Build history of the part. All positions in model axes, mm. A direction names the side the tool comes from. Coordinates: 2 decimals unless noted, no trailing zeros. Order: outer loops, then holes, each group sorted by start corner. A loop starts at its lowest first (then second) coordinate and runs counter-clockwise, first axis right, second up. Notation, with made-up numbers: (46.5, 59) - (102.5, 59) arc R21 ccw to (102.5, 95) - close; hole circle Ø3 at (-35, 7.5). An arc over 180 degrees is marked (long way). One line per item, written item: value.
from build123d import *

# Parameters (mm, degrees)
SKETCH1_W           = 40
SKETCH1_H           = 12.1
BOSS_EXTRUDE1_DEPTH = 3
SKETCH2_W           = 40
SKETCH2_H           = 3
SKETCH2_H_2         = 7
BOSS_EXTRUDE2_DEPTH = 10
SKETCH3_W           = 10.2
SKETCH3_H           = 3.2
CUT_EXTRUDE1_DEPTH  = 44.765397291
SKETCH4_W           = 4
SKETCH4_H           = 8
CUT_EXTRUDE2_DEPTH  = 20
SKETCH5_R           = 4.5
CUT_EXTRUDE3_DEPTH  = 3
FILLET2_R           = 10
FILLET1_R           = 0.4


with BuildPart() as part:
    # Sketch1 → Boss-Extrude1 (new body)
    with BuildSketch(Plane(origin=(0, 0, 0), x_dir=(1, 0, 0), z_dir=(0, 1, 0))):
        with Locations((20, -6.05)):
            Rectangle(SKETCH1_W, SKETCH1_H)
    extrude(amount=BOSS_EXTRUDE1_DEPTH)

    # Sketch2 → Boss-Extrude2 (add)
    with BuildSketch(Plane(origin=(0, 3, 0), x_dir=(1, 0, 0), z_dir=(0, 1, 0))):
        with Locations((20, -1.5)):
            Rectangle(SKETCH2_W, SKETCH2_H)
        with Locations((20, -8.6)):
            Rectangle(SKETCH2_W, SKETCH2_H_2)
    extrude(amount=BOSS_EXTRUDE2_DEPTH)

    # Sketch3 → Cut-Extrude1 (cut, through all)
    with BuildSketch(Plane(origin=(0, 0, 0), x_dir=(-1, 0, 0), z_dir=(0, 0, -1))):
        with Locations((-10, 3.6)):
            Rectangle(SKETCH3_W, SKETCH3_H)
    extrude(amount=-CUT_EXTRUDE1_DEPTH, mode=Mode.SUBTRACT)

    # Sketch4 → Cut-Extrude2 (cut)
    with BuildSketch(Plane.ZY):
        with Locations((7.1, 9)):
            Rectangle(SKETCH4_W, SKETCH4_H)
    extrude(amount=-CUT_EXTRUDE2_DEPTH, mode=Mode.SUBTRACT)

    # Sketch5 → Cut-Extrude3 (cut)
    with BuildSketch(Plane.XY.offset(12.1)):
        with Locations((9.655746404, 12.73)):
            Circle(SKETCH5_R)
    extrude(amount=-CUT_EXTRUDE3_DEPTH, mode=Mode.SUBTRACT)

    # Fillet2
    # the kernel refuses this fillet: 10 mm, written as the material it takes off along each edge
    with BuildSketch(Plane(origin=(5.163853707, 13, 9.1), x_dir=(0.32846589208199206, -0.9445158324447405, 0), z_dir=(0, 0, 1))) as fillet2_piece_1:
        with BuildLine():
            CenterArc((7.306356337, -9.231062175), FILLET2_R, 112.615500581, 41.575528471)
            Line((-1.696149814, -4.877341583), (0, 0))
            ThreePointArc((0, 0), (1.730452817, -0.346022021), (3.460905633, 0))
        make_face()
    extrude(amount=15.909634267, mode=Mode.SUBTRACT)

    # Fillet1
    fillet1_edges = [part.edges().sort_by_distance(p)[0] for p in [
        (0, 3, 4.05),
        (0, 8, 3),
        (40, 8, 3),
        (0, 13, 1.5),
        (20, 13, 3),
        (40, 13, 1.5),
        (20, 13, 0),
        (40, 3, 4.05),
        (40, 8, 5.1),
        (40, 13, 8.6),
        (30, 13, 5.1),
        (15.1, 3.6, 12.1),
        (10, 5.2, 12.1),
        (4.9, 3.6, 12.1),
        (10, 2, 12.1),
        (15.1, 3.6, 0),
        (10, 2, 0),
        (4.9, 3.6, 0),
        (20, 0, 0),
        (10, 5.2, 0),
        (40, 0, 6.05),
        (20, 0, 12.1),
        (0, 0, 6.05),
        (0, 13, 10.6),
        (0, 4, 5.1),
        (17.07381955, 13, 9.1),
        (20, 13, 7.1),
        (0, 5, 7.1),
        (0, 9, 9.1),
        (0, 6.5, 0),
        (40, 6.5, 0),
        (40, 6.5, 12.1),
        (0, 6.5, 12.1),
        (27.07381955, 13, 12.1),
        (14.147639101, 13, 10.6),
        (11.38619922, 8.576022021, 12.1),
        (3.450117075, 11.943404417, 12.1),
    ]]
    fillet(fillet1_edges, radius=FILLET1_R)


solid = part.part
1. Probe line 1 along X through (y, z) = (4, 7.75); line 2 along Z through (x, y) = (23.5, 10); line 3 along Z through (x, y) = (6, 6.5). List the from-to ranges inside material, lowest first.
Values found:
line 1: x = 0 to 4.9, 15.1 to 40
line 2: z = 0 to 3, 5.1 to 12.1
line 3: z = 0 to 3, 9.1 to 12.1
2. Band-saw the part on D-D, the plane z = 11.25. Give the cut face in (x, y).
Values found:
outline: (0, 0.4) arc R0.4 ccw to (0.4, 0) - (39.6, 0) arc R0.4 ccw to (40, 0.4) - (40, 12.6) arc R0.4 ccw to (39.6, 13) - (14.55, 13) arc R0.4 ccw to (14.15, 12.61) arc R4.5 cw to (6.3, 9.73) arc R10 ccw to (0.46, 12.93) arc R0.4 ccw to (0, 12.54) - close; hole (4.9, 2) - (15.1, 2) - (15.1, 5.2) - (4.9, 5.2) - close
3. Band-saw the part on A-A, the plane y = 7. Give the cut face in (x, z).
Values found:
outline: (0, 0.4) arc R0.4 ccw to (0.4, 0) - (39.6, 0) arc R0.4 ccw to (40, 0.4) - (40, 2.6) arc R0.4 ccw to (39.6, 3) - (0.4, 3) arc R0.4 ccw to (0, 2.6) - close; (0, 9.5) arc R0.4 ccw to (0.4, 9.1) - (20, 9.1) - (20, 5.1) - (39.6, 5.1) arc R0.4 ccw to (40, 5.5) - (40, 11.7) arc R0.4 ccw to (39.6, 12.1) - (0.4, 12.1) arc R0.4 ccw to (0, 11.7) - close
4. Band-saw the part on B-B, the plane z = 4. Give the cut face in (x, y).
Values found:
outline: (0, 0.4) arc R0.4 ccw to (0.4, 0) - (39.6, 0) arc R0.4 ccw to (40, 0.4) - (40, 2.6) arc R0.4 ccw to (39.6, 3) - (15.1, 3) - (15.1, 2) - (4.9, 2) - (4.9, 3) - (0.4, 3) arc R0.4 ccw to (0, 2.6) - close
5. Band-saw the part on C-C, the plane x = 16.5. Give the cut face in (y, z).
Values found:
outline: (0, 0.4) arc R0.4 ccw to (0.4, 0) - (12.6, 0) arc R0.4 ccw to (13, 0.4) - (13, 2.6) arc R0.4 ccw to (12.6, 3) - (3, 3) - (3, 5.1) - (5, 5.1) - (5, 9.1) - (12.6, 9.1) arc R0.4 ccw to (13, 9.5) - (13, 11.7) arc R0.4 ccw to (12.6, 12.1) - (0.4, 12.1) arc R0.4 ccw to (0, 11.7) - close
6. 3-axis set-ups, long thin cutter, end or side, ignore diameter. For faces 1 (the face through (3.7, 11.81, 10.38)), 2 (the face through (10, 5.2, 10)), 3 (the face through (30, 8, 5.1)): which of +Z, -Z, +X, -X, +Y, -Y reach the whole face in a straight line?
Values found:
face 1: +Z, +Y
face 2: +Z, -Z
face 3: +X, -X, +Y
7. Two-plate mould, pull along X, no slides. Class faces 4 (the face through (10, 2, 6)), 5 (the face through (20, 9, 7)), 6 (the face through (11.13, 8.48, 10.42)), 7 (the face through (3, 5, 7)): pulls with the +X half, pulls with the -X half, needs draft (parallel to the pull), parting line crosses it, or undercut.
Values found:
face 4: undercut
face 5: pulls with the -X half
face 6: undercut
face 7: needs draft
8. Flat gauge pins, fed straight in: P1, Ø3, axis at x = 18, z = 7.5, coming from the +Y side; P2, Ø2, axis at y = 10.5, z = 8, coming from the -X side; P3, Ø0.6, axis at x = 25.5, z = 4, coming from the +Y side. Where does each tip first touch, or does it go through?
Values found:
P1: stops at y = 5
P2: stops at x = 20
P3: stops at y = 3
